Here's how the part is built. I have some questions about the finished solid (model axes, mm). Face numbers are marked on the shaded views. Round coordinates to 2 decimals unless told otherwise and drop trailing zeros. Loops run counter-clockwise (first coordinate to the right, second up) from the corner with the lowest first, then second, coordinate; pieces in that order, holes last. Notation, with made-up numbers: M 15,28 L 22,28 A14 cw 22,34 Z; hole C 49.25,17.25 d9. An arc over 180 degrees is marked long. Use a Markdown table: item, result.
```python
from build123d import *

# Parameters (mm, degrees)
BASE_FLANGE1_DEPTH               = 3.175
EDGE_FLANGE1_STRIP_W             = 19.05
EDGE_FLANGE1_STRIP_H             = 3.175
EDGE_FLANGE1_STRIP_CUT_DEPTH     = 654.05
EDGE_FLANGE1_DEPTH               = 654.05
EDGE_FLANGE2_START               = 4.7625
EDGE_FLANGE2_DEPTH               = 644.525
EDGE_FLANGE2_START_2             = 3.175
EDGE_FLANGE2_2_OUTLINE_W         = 1.5875
EDGE_FLANGE2_2_OUTLINE_H         = 3.175
EDGE_FLANGE2_2_DEPTH             = 1.5875
EDGE_FLANGE2_START_3             = 649.2875
EDGE_FLANGE2_3_OUTLINE_W         = 1.5875
EDGE_FLANGE2_3_OUTLINE_H         = 3.175
EDGE_FLANGE2_3_DEPTH             = 1.5875
EDGE_FLANGE2_4_DEPTH             = 644.525
F_17_64_0_26563_DIAMETER_HOLE1_D = 6.746875
LPATTERN1_COUNT                  = 7
LPATTERN1_PITCH                  = 101.6


# Read off the part's stored shape, not the designer's step: Edge-Flange2
# Sheet-metal steps are written as plain solids
with BuildPart() as part:
    # Sketch2 → Base-Flange1 (new body)
    with BuildSketch(Plane.XY):
        Polygon((4.7625, 0), (4.7625, 6.35), (0, 6.35), (0, 38.1), (654.05, 38.1), (654.05, 6.35), (649.2875, 6.35), (649.2875, 0), align=None)
    extrude(amount=-BASE_FLANGE1_DEPTH)

    # Edge-Flange1 strip (across the edge) → Edge-Flange1 strip cut (cut)
    with BuildSketch(Plane(origin=(0, 38.1, -3.175), x_dir=(0, -1, 0), z_dir=(1, 0, 0))):
        with Locations((-3.175, -1.5875)):
            Rectangle(EDGE_FLANGE1_STRIP_W, EDGE_FLANGE1_STRIP_H)
    extrude(amount=EDGE_FLANGE1_STRIP_CUT_DEPTH, mode=Mode.SUBTRACT)

    # Edge-Flange1 section (across the edge) → Edge-Flange1 (add)
    with BuildSketch(Plane(origin=(0, 38.1, -3.175), x_dir=(0, -1, 0), z_dir=(1, 0, 0))):
        with BuildLine():
            Line((0, 3.175), (0, 34.925))
            Line((0, 34.925), (3.175, 34.925))
            Line((3.175, 34.925), (3.175, 3.175))
            ThreePointArc((3.175, 3.175), (4.10493597, 0.92993597), (6.35, 0))
            Line((6.35, 0), (6.35, -3.175))
            ThreePointArc((6.35, -3.175), (1.859871939, -1.315128061), (0, 3.175))
        make_face()
    extrude(amount=EDGE_FLANGE1_DEPTH)

    # Edge-Flange2 outline → Edge-Flange2 (cut)
    with BuildSketch(Plane.YZ.offset(EDGE_FLANGE2_START)):
        with BuildLine():
            Line((0, -3.175), (0.850738685, -3.175))
            ThreePointArc((0.850738685, -3.175), (3.174999999, -0.850738686), (6.35, 0))
            Line((6.35, 0), (0, 0))
            Line((0, 0), (0, -3.175))
        make_face()
    extrude(amount=EDGE_FLANGE2_DEPTH, mode=Mode.SUBTRACT)

    # Edge-Flange2 2 outline → Edge-Flange2 2 (cut)
    with BuildSketch(Plane.YZ.offset(EDGE_FLANGE2_START_2)):
        with Locations((7.14375, -1.5875)):
            Rectangle(EDGE_FLANGE2_2_OUTLINE_W, EDGE_FLANGE2_2_OUTLINE_H)
    extrude(amount=EDGE_FLANGE2_2_DEPTH, mode=Mode.SUBTRACT)

    # Edge-Flange2 3 outline → Edge-Flange2 3 (cut)
    with BuildSketch(Plane.YZ.offset(EDGE_FLANGE2_START_3)):
        with Locations((7.14375, -1.5875)):
            Rectangle(EDGE_FLANGE2_3_OUTLINE_W, EDGE_FLANGE2_3_OUTLINE_H)
    extrude(amount=EDGE_FLANGE2_3_DEPTH, mode=Mode.SUBTRACT)

    # Edge-Flange2 4 outline → Edge-Flange2 4 (add)
    with BuildSketch(Plane.YZ.offset(EDGE_FLANGE2_START)):
        with BuildLine():
            Line((0, -38.1), (3.175, -38.1))
            Line((3.175, -38.1), (3.175, -6.35))
            ThreePointArc((3.175, -6.35), (4.10493597, -4.10493597), (6.35, -3.175))
            Line((6.35, -3.175), (0.850738685, -3.175))
            ThreePointArc((0.850738685, -3.175), (0.216371003, -4.706499064), (0, -6.35))
            Line((0, -6.35), (0, -38.1))
        make_face()
    extrude(amount=EDGE_FLANGE2_4_DEPTH)

    # 17/64 (0.26563) Diameter Hole1 (through all)
    with Locations(Plane.XY):
        with Locations((22.352, 22.225)):
            f_17_64_0_26563_diameter_hole1 = Hole(F_17_64_0_26563_DIAMETER_HOLE1_D / 2)

    # LPattern1: 17/64 (0.26563) Diameter Hole1 ×7
    with Locations(*[(i * LPATTERN1_PITCH, 0, 0) for i in range(1, LPATTERN1_COUNT)]):
        add(f_17_64_0_26563_diameter_hole1, mode=Mode.SUBTRACT)


solid = part.part
```
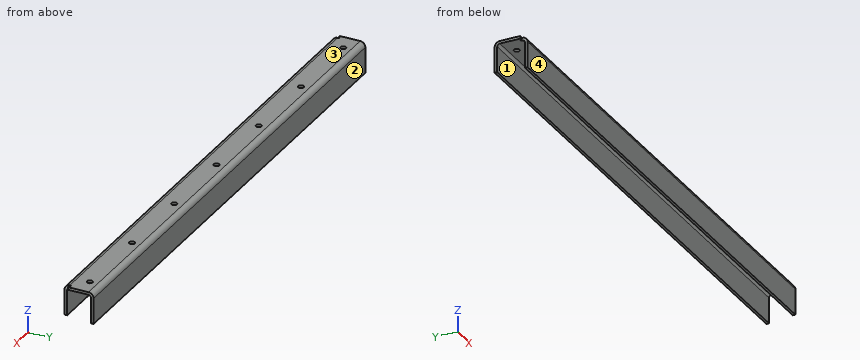
Q1. We'd pull the mould along Y, two halves only. Please class the marked faces 1, 2, 3 and 4: pulls with the +Y half, pulls with the -Y half, needs draft (parallel to the pull), parting line crosses it, or undercut.
Return value:
| item | result |
|---|---|
| face 1 | undercut |
| face 2 | pulls with the +Y half |
| face 3 | needs draft |
| face 4 | pulls with the -Y half |
Q2. I need wall thicknesses on line 1 (Y direction, x = 356.5, z = -35.5) (3 decimals); line 2 (Y direction, x = 275.5, z = -5.5); line 3 (Z direction, x = 530, y = 6.5) (3 decimals). Which ranges of each line are inside material? Lowest first, please. Write a range as from..to.
Return value:
| item | result |
|---|---|
| line 1 | y = 0..3.175, 34.925..38.1 |
| line 2 | y = 0.06..3.29, 34.81..38.04 |
| line 3 | z = -3.175..0 |
Q3. Imagine slicing it at B-B, the plane x = 374.5. Please give me the cut outline in (y, z) (3 decimals), then the cut area to 3 significant figures.
Return value:
| item | result |
|---|---|
| outline | M 0,-38.1 L 3.175,-38.1 L 3.175,-6.35 A3.175 cw 6.35,-3.175 L 31.75,-3.175 A3.175 cw 34.925,-6.35 L 34.925,-38.1 L 38.1,-38.1 L 38.1,-6.35 A6.35 ccw 31.75,0 L 6.35,0 A6.35 ccw 0,-6.35 Z |
| area | 330 mm^2 |
Q4. Will these pins go through, and if not, where does the flat tip stop? P1, Ø1.6, axis at x = 2.5, z = -1, coming from the -Y side; P2, Ø7.5, axis at x = 413.5, y = 24.5, coming from the -Z side (3 decimals); P3, Ø2.5, axis at y = 4.5, z = -10.5, coming from the -X side; P4, Ø0.8, axis at x = 4.5, z = -1.5, coming from the -Y side.
Return value:
| item | result |
|---|---|
| P1 | stops at y = 6.35 |
| P2 | stops at z = -3.175 |
| P3 | passes through |
| P4 | stops at y = 1.92 |
